from build123d import *

# Parameters (mm, degrees)
F3_DEPTH = 13
F3_TAPER = 12
F1_W     = 3.75
F1_H     = 9
F2_DEPTH = 5


with BuildPart() as f3:
    # F0 (on Front) → F3 (new body)
    with BuildSketch(Plane.XZ):
        with BuildLine():
            ThreePointArc((0, 4), (1.1715728753, 1.1715728753), (4, 0))
            Line((4, 0), (56, 0))
            ThreePointArc((56, 0), (58.8284271247, 1.1715728753), (60, 4))
            Line((60, 4), (60, 91))
            ThreePointArc((60, 91), (58.8284271247, 93.8284271247), (56, 95))
            Line((56, 95), (4, 95))
            ThreePointArc((4, 95), (1.1715728753, 93.8284271247), (0, 91))
            Line((0, 91), (0, 4))
        make_face()
    extrude(amount=F3_DEPTH, taper=F3_TAPER)

    # F1 (on face) → F2 (cut)
    with BuildSketch(Plane(origin=(57.4063637293, -12.2020992923, 0), x_dir=(0.2079116908, 0.9781476007, 0), z_dir=(0.9781476007, -0.2079116908, 0))):
        with Locations((5.8294875824, 19)):
            Rectangle(F1_W, F1_H)
    extrude(amount=-F2_DEPTH, mode=Mode.SUBTRACT)


solid = f3.part
The listing builds one solid part. Answer for the finished solid, in the listing's coordinates (mm). A direction names the side the tool comes from. Round coordinates to 2 decimals unless told otherwise and drop trailing zeros. Use a Markdown table: item, result. Add a question column.
1. Flat-ended cylindrical pins translate along their axes: P1, Ø5, axis at x = 56, y = -5, coming from the -Z side; P2, Ø6, axis at x = 7.5, y = -6, coming from the -Z side; P3, Ø2, axis at y = -3, z = 23, coming from the -X side. Find the tip coordinate at first contact, or state that the pin passes through.
2. A tool of negligible diameter and unlimited length cuts with its end or side. For faces 4 (the face through (55.817, -7.822, 18.937)), 5 (the face through (56, -6, 23.5)), 6 (the face through (2.142, -6.591, 2.183)), from which of +Z, -Z, +X, -X, +Y, -Y can it reach the whole face along a straight path? Write none if from no direction.
3. Consider line 1 (Z direction, x = 48.5, y = -4.75); line 2 (X direction, y = -9.75, z = 60.5); line 3 (X direction, y = -8.5, z = 5). Determine where each line is inside the solid, lowest interval first.
4. For a pull along Y with two mould halves and no side action, classify faces 1 (the face through (57.858, -6.591, 92.817)), 2 (the face through (56.597, -4.153, 18.937)), 3 (the face through (30, 0, 47)) as +Y half, -Y half, draft (parallel to the pull), parting line (faces both ways), or undercut.
Reported:
| question | item | result |
|---|---|---|
| 1 | P1 | z = 0.53 |
| 1 | P2 | z = 0.64 |
| 1 | P3 | x = 0.43 |
| 2 | face 4 | +X |
| 2 | face 5 | none |
| 2 | face 6 | -Z, -X, -Y |
| 3 | line 1 | 1.01 to 93.99 |
| 3 | line 2 | 2.07 to 57.93 |
| 3 | line 3 | 1.81 to 58.19 |
| 4 | face 1 | -Y half |
| 4 | face 2 | undercut |
| 4 | face 3 | +Y half |
